Here's how the part is built. I have some questions about the finished solid (model axes, mm). Face numbers are marked on the shaded views. Round coordinates to 2 decimals unless told otherwise and drop trailing zeros. Order: outer loops, then holes, each group sorted by start corner. A loop starts at its lowest first (then second) coordinate and runs counter-clockwise, first axis right, second up.
```python
from build123d import *

# Parameters (mm, degrees)
SZKIC1_W                        = 6
SZKIC1_H                        = 40
SZKIC2_W                        = 18
SZKIC2_H                        = 8
WYTNIJ_WYCI_GNI_CIE1_DEPTH      = 20
WYTNIJ_WYCI_GNI_CIE2_DEPTH      = 42.976183724
WYTNIJ_WYCI_GNI_CIE2_DEPTH_BACK = 42.976183724
SZKIC3_R                        = 4
WYTNIJ_WYCI_GNI_CIE3_START      = 6
SZKIC3_4_R                      = 6
SZKIC3_4_R_2                    = 4
WYTNIJ_WYCI_GNI_CIE3_DEPTH      = 36.976183767


with BuildPart() as part:
    # Szkic1 → Obr_t1 (revolve)
    with BuildSketch(Plane(origin=(0, 0, 0), x_dir=(1, 0, 0), z_dir=(0, 1, 0))):
        with Locations((3, 20)):
            Rectangle(SZKIC1_W, SZKIC1_H)
        Polygon((0, 0), (0, -25), (9, -25), (9, 0), (6, 0), align=None)
    revolve(axis=Axis((0, 0, 44.409951059), (0, 0, -1)))

    # Szkic2 → Wytnij-wyci_gni_cie1 (cut)
    with BuildSketch(Plane.XY.offset(25)):
        Rectangle(SZKIC2_W, SZKIC2_H)
    extrude(amount=-WYTNIJ_WYCI_GNI_CIE1_DEPTH, mode=Mode.SUBTRACT)

    # Szkic3 → Wytnij-wyci_gni_cie2 (cut, two sides: drawn at the far end of the back side and taken through both)
    with BuildSketch(Plane(origin=(0, 0, 0), x_dir=(1, 0, 0), z_dir=(0, 1, 0)).offset(-WYTNIJ_WYCI_GNI_CIE2_DEPTH_BACK)):
        with Locations(Location((0, -15, 0), (0, 0, 270))):
            Circle(SZKIC3_R)
    extrude(amount=WYTNIJ_WYCI_GNI_CIE2_DEPTH + WYTNIJ_WYCI_GNI_CIE2_DEPTH_BACK, mode=Mode.SUBTRACT)

    # Szkic3_4 → Wytnij-wyci_gni_cie3 (cut, through all)
    with BuildSketch(Plane(origin=(0, 0, 0), x_dir=(1, 0, 0), z_dir=(0, 1, 0)).offset(WYTNIJ_WYCI_GNI_CIE3_START)):
        with Locations(Location((0, -15, 0), (0, 0, 90))):
            Circle(SZKIC3_4_R)
        with Locations(Location((0, -15, 0), (0, 0, 270))):
            Circle(SZKIC3_4_R_2, mode=Mode.SUBTRACT)
    extrude(amount=WYTNIJ_WYCI_GNI_CIE3_DEPTH, mode=Mode.SUBTRACT)


solid = part.part
```
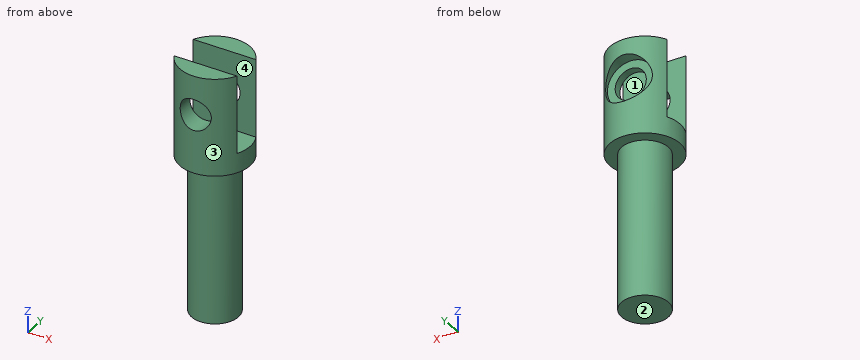
1. I'm going to push flat-ended pins straight in: P1, Ø8, axis at y = 1, z = 9.5, coming from the -X side; P2, Ø3, axis at x = 4, y = -5, coming from the -Z side; P3, Ø10, axis at y = 0, z = -32.5, coming from the +X side; P4, Ø1, axis at x = 3.5, z = -1, coming from the -Y side. Where does each tip first touch, or does it pass through?
Evaluation:
P1: stops at x = -8.06
P2: stops at z = -40
P3: stops at x = 6
P4: stops at y = -5.2
2. If we mould it in two halves opening along Y, with no side actions, what happens to the marked faces 1, 2, 3 and 4? For each: released by +Y, released by -Y, zero draft, split by the parting line, or undercut.
Evaluation:
face 1: undercut
face 2: zero draft
face 3: split by the parting line
face 4: undercut
3. If we section it at C-C, the plane x = 0: Write out the boundary of the cut face in (y, z), and give its area (3 significant figures).
Evaluation:
outline: (-9, 0) - (-6, 0) - (-6, -40) - (6, -40) - (6, 0) - (9, 0) - (9, 9) - (6, 9) - (6, 11) - (4, 11) - (4, 5) - (-4, 5) - (-4, 11) - (-9, 11) - close; (-9, 19) - (-4, 19) - (-4, 25) - (-9, 25) - close; (4, 19) - (6, 19) - (6, 21) - (9, 21) - (9, 25) - (4, 25) - close
area: 678 mm2
4. I need wall thicknesses on probe 1 along Z at (x, y) = (0, 5.5); probe 2 along Y at (x, z) = (4, 18); probe 3 along Z at (x, y) = (0, -6.2). Which ranges of each line are inside material? Lowest first, please.
Evaluation:
probe 1: z = -40 to 11, 19 to 25
probe 2: y = -8.06 to -4, 4 to 6
probe 3: z = 0 to 11, 19 to 25
5. If we section it at A-A, the plane y = 0: Write out the boundary of the cut face in (x, z).
Evaluation:
outline: (-9, 0) - (-6, 0) - (-6, -40) - (6, -40) - (6, 0) - (9, 0) - (9, 5) - (-9, 5) - close
6. If we section it at B-B, the plane z = 15: Write out the boundary of the cut face in (x, y).
Evaluation:
outline: (-8.06, -4) arc R9 ccw to (-4, -8.06) - (-4, -4) - close; (-8.06, 4) - (-4, 4) - (-4, 6) - (-6, 6) - (-6, 6.71) arc R9 ccw to start; (4, -8.06) arc R9 ccw to (8.06, -4) - (4, -4) - close; (4, 4) - (8.06, 4) arc R9 ccw to (6, 6.71) - (6, 6) - (4, 6) - close
7. If we section it at D-D, the plane x = 7.5: Write out the boundary of the cut face in (y, z), and give its area (3 significant figures).
Evaluation:
outline: (-4.97, 0) - (4.97, 0) - (4.97, 25) - (4, 25) - (4, 5) - (-4, 5) - (-4, 25) - (-4.97, 25) - close
area: 88.7 mm2
